from build123d import *

# Parameters (mm, degrees)
F1_R     = 2.25
F1_R_2   = 1.75
F1_R_3   = 3
F2_DEPTH = 3
F3_W     = 17
F3_H     = 35
F4_DEPTH = 3.001
F5_R     = 4


with BuildPart() as f2:
    # F1 (on Top) → F2 (new body)
    with BuildSketch(Plane.XY):
        Polygon((44.55, 58.5), (-32.5, 58.5), (-45.55, 58.5), (-45.55, 37.5), (-32.5, 37.5), (-32.5, 0), (-32.5, -58.5), (44.55, -58.5), (44.55, -37.55), (55.5, -37.55), (55.5, 37.55), (44.55, 37.55), align=None)
        with Locations((0, -45)):
            Circle(F1_R, mode=Mode.SUBTRACT)
        with Locations((-8.9, -33.5)):
            Circle(F1_R_2, mode=Mode.SUBTRACT)
        with Locations((25.5, -33.5)):
            Circle(F1_R_2, mode=Mode.SUBTRACT)
        with Locations((37.5, -45)):
            Circle(F1_R, mode=Mode.SUBTRACT)
        with Locations((30.5, -15)):
            Circle(F1_R_3, mode=Mode.SUBTRACT)
        with Locations((-37.5, 45)):
            Circle(F1_R, mode=Mode.SUBTRACT)
        with Locations((-8.9, 51.5)):
            Circle(F1_R_2, mode=Mode.SUBTRACT)
        with Locations((0, 45)):
            Circle(F1_R, mode=Mode.SUBTRACT)
        with Locations((30.5, 15)):
            Circle(F1_R_3, mode=Mode.SUBTRACT)
        with Locations((25.5, 51.5)):
            Circle(F1_R_2, mode=Mode.SUBTRACT)
        with Locations((37.5, 45)):
            Circle(F1_R, mode=Mode.SUBTRACT)
    extrude(amount=F2_DEPTH)

    # F3 (on Top) → F4 (cut, through all)
    with BuildSketch(Plane.XY):
        with Locations((-24, -41)):
            Rectangle(F3_W, F3_H)
    extrude(amount=F4_DEPTH, mode=Mode.SUBTRACT)

    # F5
    f5_edges = [f2.edges().sort_by_distance(p)[0] for p in [
        (-45.55, 37.5, 1.5),
        (-45.55, 58.5, 1.5),
        (-32.5, 37.5, 1.5),
        (-32.5, -23.5, 1.5),
        (-15.5, -58.5, 1.5),
        (-15.5, -23.5, 1.5),
        (44.55, -58.5, 1.5),
        (44.55, -37.55, 1.5),
        (55.5, -37.55, 1.5),
        (55.5, 37.55, 1.5),
        (44.55, 37.55, 1.5),
        (44.55, 58.5, 1.5),
    ]]
    fillet(f5_edges, radius=F5_R)


solid = f2.part
Model file for the job. Use its own axes, mm. A direction names the side the tool comes from. Give positions to 0.01 mm unless a question says otherwise; leave off trailing zeros. Write each loop counter-clockwise with the first axis right and the second up, starting at its lowest first coordinate (ties: lowest second). Pieces come first, ordered by that corner, then holes. Notation, with made-up numbers: (39, 1) - (83, 1) arc R23 cw to (83, 23) - close; hole circle Ø2 at (41.5, 22.5). An arc over 180 degrees is marked (long way). Answer as CSV lines item,"result".
1. 3-axis set-ups, long thin cutter, end or side, ignore diameter. For faces 1 (the face through (23.75, -33.42, 1.48)), 2 (the face through (50, -37.55, 1)), 3 (the face through (-15.5, -41, 1)): which of +Z, -Z, +X, -X, +Y, -Y reach the whole face in a straight line?
Responses:
face 1,"+Z, -Z"
face 2,"+Z, -Z, +X, -Y"
face 3,"+Z, -Z, -X, -Y"
2. Drill centre lines: L1, parallel to Y at x = 0, z = 2.4; L2, parallel to Y at x = 25.5, z = 1; L3, parallel to X at y = 22, z = 1.9. Where is each one in solid material? Low to high. Write a range as [from, to].
Responses:
L1,"y = [-58.5, -47.25], [-42.75, 42.75], [47.25, 58.5]"
L2,"y = [-58.5, -35.25], [-31.75, 49.75], [53.25, 58.5]"
L3,"x = [-32.5, 55.5]"
3. Band-saw the part on A-A (x = -8.9). Write the cut outline in (y, z).
Responses:
outline,"(-58.5, 0) - (-35.25, 0) - (-35.25, 3) - (-58.5, 3) - close; (-31.75, 0) - (49.75, 0) - (49.75, 3) - (-31.75, 3) - close; (53.25, 0) - (58.5, 0) - (58.5, 3) - (53.25, 3) - close"
4. Band-saw the part on B-B (y = -15). Write the cut outline in (x, z).
Responses:
outline,"(-32.5, 0) - (27.5, 0) - (27.5, 3) - (-32.5, 3) - close; (33.5, 0) - (55.5, 0) - (55.5, 3) - (33.5, 3) - close"
5. Band-saw the part on C-C (z = 2.45). Count the separate pieces of the cut face and the enclosed holes in it, and give its area (3 significant figures).
Responses:
separate pieces,"1"
enclosed holes,"11"
area,"9,330 mm2"
6. Two-plate mould, pull along X, no slides. Class faces 4 (the face through (44.55, 48, 1)), 5 (the face through (-33.703, 36.359, 1.521)), 6 (the face through (50, 37.55, 1)), 7 (the face through (-37.79, 47.23, 1.48)): +X half, -X half, draft (parallel to the pull), parting line (faces both ways), or undercut.
Responses:
face 4,"+X half"
face 5,"-X half"
face 6,"draft"
face 7,"undercut"
7. Band-saw the part on D-D (y = 0.5). Write the cut outline in (x, z).
Responses:
outline,"(-32.5, 0) - (55.5, 0) - (55.5, 3) - (-32.5, 3) - close"
8. Pin check, flat tips, straight feed: pin 1 (0.9 mm diameter, centred on y = 47, z = 2, fed in from +X); pin 2 (0.9 mm diameter, centred on y = 4.5, z = 1, fed in from -X); pin 3 (2.5 mm diameter, centred on x = 37.5, y = -45, fed in from +Z); pin 4 (0.9 mm diameter, centred on y = -44.5, z = 2, fed in from -X). Stop position of each tip, or through.
Responses:
pin 1,"stops at x = 44.55"
pin 2,"stops at x = -32.5"
pin 3,"passes through"
pin 4,"stops at x = -15.5"
